Source: CAD feature listing. Evaluate the final solid. Frame: model axes, mm. A direction names the side the tool comes from. Round coordinates to 2 decimals unless told otherwise and drop trailing zeros. Loops run counter-clockwise (first coordinate to the right, second up) from the corner with the lowest first, then second, coordinate; pieces in that order, holes last. Notation, with made-up numbers: (-15.75, 28) - (2.25, 28) arc R33 ccw to (2.25, 64) - close; hole circle Ø9 at (17.25, 7). An arc over 180 degrees is marked (long way). One line per question, with ' | ' between items.
from build123d import *

# Parameters (mm, degrees)
SKETCH2_W                                       = 101.6
SKETCH2_H                                       = 38.1
BOSS_EXTRUDE1_DEPTH                             = 12.7
SKETCH3_W                                       = 25.4
SKETCH3_H                                       = 3.302
CUT_EXTRUDE1_DEPTH                              = 65.757547823
BOSS_EXTRUDE2_DEPTH                             = 12.7
CBORE_FOR_0_PAN_HEAD_MACHINE_SCREW1_D           = 6.858
CBORE_FOR_0_PAN_HEAD_MACHINE_SCREW1_CBORE_D     = 19.05
CBORE_FOR_0_PAN_HEAD_MACHINE_SCREW1_CBORE_DEPTH = 4.826
FILLET1_R                                       = 6.35


with BuildPart() as part:
    # Sketch2 → Boss-Extrude1 (new body)
    with BuildSketch(Plane(origin=(0, 0, 0), x_dir=(1, 0, 0), z_dir=(0, 1, 0))):
        Rectangle(SKETCH2_W, SKETCH2_H)
    extrude(amount=BOSS_EXTRUDE1_DEPTH)

    # Sketch3 → Cut-Extrude1 (cut, through all)
    with BuildSketch(Plane.XY.offset(19.05)):
        with Locations((0, 1.651)):
            Rectangle(SKETCH3_W, SKETCH3_H)
    extrude(amount=-CUT_EXTRUDE1_DEPTH, mode=Mode.SUBTRACT)

    # Sketch5 → Boss-Extrude2 (add)
    with BuildSketch(Plane.XY.offset(19.05)):
        with BuildLine():
            Line((-19.05, 12.7), (19.05, 12.7))
            Line((19.05, 12.7), (19.05, 38.1))
            ThreePointArc((19.05, 38.1), (0, 57.15), (-19.05, 38.1))
            Line((-19.05, 38.1), (-19.05, 12.7))
        make_face()
    extrude(amount=-BOSS_EXTRUDE2_DEPTH)

    # CBORE for #0 Pan Head Machine Screw1 (through all)
    with Locations(Plane.XY.offset(19.05)):
        with Locations((0, 38.1)):
            CounterBoreHole(CBORE_FOR_0_PAN_HEAD_MACHINE_SCREW1_D / 2, CBORE_FOR_0_PAN_HEAD_MACHINE_SCREW1_CBORE_D / 2, CBORE_FOR_0_PAN_HEAD_MACHINE_SCREW1_CBORE_DEPTH)

    # Fillet1
    fillet1_edges = [part.edges().sort_by_distance(p)[0] for p in [
        (-50.8, 6.35, -19.05),
        (50.8, 6.35, -19.05),
        (50.8, 6.35, 19.05),
        (-50.8, 6.35, 19.05),
    ]]
    fillet(fillet1_edges, radius=FILLET1_R)


solid = part.part
1. Section query B-B, the plane z = 11. Return loops of the section in (x, y), plus the area to 3 significant figures.
Worked out:
outline: (-50.8, 0) - (-12.7, 0) - (-12.7, 3.3) - (12.7, 3.3) - (12.7, 0) - (50.8, 0) - (50.8, 12.7) - (19.05, 12.7) - (19.05, 38.1) arc R19.05 ccw to (-19.05, 38.1) - (-19.05, 12.7) - (-50.8, 12.7) - close; hole circle Ø6.86 at (0, 38.1) | area: 2,710 mm2
2. Contact query for flat-ended pins moving along their axis: P1, Ø12, axis at x = -2.5, z = -14.5, coming from the -Y side; P2, Ø14, axis at y = 31, z = 14, coming from the +X side; P3, Ø8, axis at x = 0, y = 38.1, coming from the +Z side. Output: stop coordinate, or through.
Worked out:
P1: stops at y = 3.3 | P2: stops at x = 19.05 | P3: stops at z = 14.22
3. Section query A-A, the plane x = 0. Return loops of the section in (y, z) (3 decimals), plus the area to 3 significant figures.
Worked out:
outline: (3.302, -19.05) - (12.7, -19.05) - (12.7, 6.35) - (34.671, 6.35) - (34.671, 14.224) - (28.575, 14.224) - (28.575, 19.05) - (3.302, 19.05) - close; (41.529, 6.35) - (57.15, 6.35) - (57.15, 19.05) - (47.625, 19.05) - (47.625, 14.224) - (41.529, 14.224) - close | area: 777 mm2
4. Section query D-D, the plane y = 25. Return loops of the section in (x, z), plus the area to 3 significant figures.
Worked out:
outline: (-19.05, 6.35) - (19.05, 6.35) - (19.05, 19.05) - (-19.05, 19.05) - close | area: 484 mm2
5. Mould query, pull axis Y, two halves, no side actions, for faces 1 (the cylindrical face through (-1.24, 47.544, 16.671)), 2 (the flat face through (-50.8, 6, 0)), 3 (the flat face through (0, 3.302, 0)). Classes: released by +Y, released by -Y, zero draft, split by the parting line, or undercut.
Worked out:
face 1: undercut | face 2: zero draft | face 3: released by -Y
6. Access query for faces 4 (the flat face through (19.05, 25, 13)), 5 (the flat face through (-12.7, 2, 0)), 6 (the flat face through (-19.05, 26, 13)), 7 (the flat face through (-1, 12.7, 0)), 8 (the flat face through (4, 38, 14.224)). Directions: +Z, -Z, +X, -X, +Y, -Y. A direction counts if a zero-diameter tool reaches every point of the face in a straight line with its end or side. Return the directions, or none.
Worked out:
face 4: +Z, -Z, +X, +Y | face 5: +Z, -Z, -Y | face 6: +Z, -Z, -X, +Y | face 7: -Z, +Y | face 8: +Z
7. Material intervals for probe 1 along Y at (x, z) = (0, 8.5); probe 2 along X at (y, z) = (38, 8); probe 3 along Y at (x, z) = (0, 16) (3 decimals), sorted ascending.
Worked out:
probe 1: y = 3.3 to 34.67, 41.53 to 57.15 | probe 2: x = -19.05 to -3.43, 3.43 to 19.05 | probe 3: y = 3.302 to 28.575, 47.625 to 57.15
8. Section query C-C, the plane z = -5. Return loops of the section in (x, y), plus the area to 3 significant figures.
Worked out:
outline: (-50.8, 0) - (-12.7, 0) - (-12.7, 3.3) - (12.7, 3.3) - (12.7, 0) - (50.8, 0) - (50.8, 12.7) - (-50.8, 12.7) - close | area: 1,210 mm2
